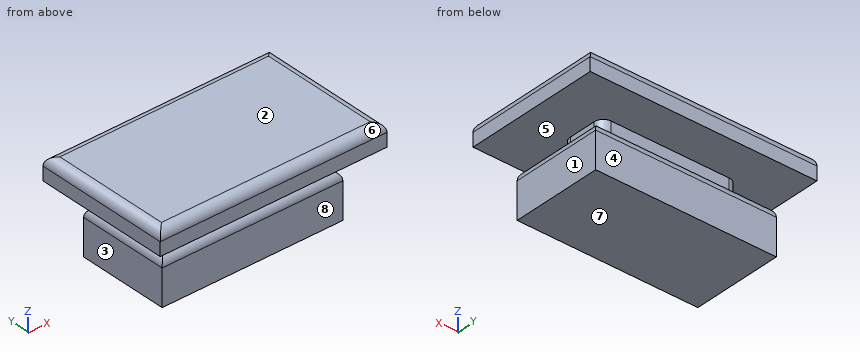
from build123d import *

# Parameters (mm, degrees)
F0_W     = 101.5923656523
F0_H     = 51.0535798967
F1_DEPTH = 25.4
F2_R     = 5.08
F3_W     = 76.4648839831
F3_H     = 25.6656967103
F4_DEPTH = 12.7
F5_R     = 5.08
F6_W     = 127.4997331202
F6_H     = 76.2346722186
F7_DEPTH = 12.7
F8_R     = 5.08


with BuildPart() as f1:
    # F0 (on Top) → F1 (new body)
    with BuildSketch(Plane.XY):
        with Locations((-14.3452938646, -5.9895161539)):
            Rectangle(F0_W, F0_H)
    extrude(amount=F1_DEPTH)

    # F2
    f2_edges = [f1.edges().sort_by_distance(p)[0] for p in [
        (-14.345294, -31.516306, 25.4),
        (-65.141477, -5.989516, 25.4),
        (-14.345294, 19.537274, 25.4),
        (36.450889, -5.989516, 25.4),
    ]]
    fillet(f2_edges, radius=F2_R)

    # F3 (on face) → F4 (join)
    with BuildSketch(Plane.XY.offset(25.4)):
        with Locations((-14.4407190382, -3.7901271135)):
            Rectangle(F3_W, F3_H)
    extrude(amount=F4_DEPTH)

    # F5
    f5_edges = [f1.edges().sort_by_distance(p)[0] for p in [
        (-52.673161, -16.622975, 31.75),
        (23.791723, -16.622975, 31.75),
        (-52.673161, 9.042721, 31.75),
        (23.791723, 9.042721, 31.75),
    ]]
    fillet(f5_edges, radius=F5_R)

    # F6 (on face) → F7 (join)
    with BuildSketch(Plane.XY.offset(38.1)):
        with Locations((-13.627236709, -6.3019637018)):
            Rectangle(F6_W, F6_H)
        with BuildLine():
            Line((-47.5931610298, 9.0427212417), (18.7117229533, 9.0427212417))
            ThreePointArc((18.7117229533, 9.0427212417), (22.3038254017, 7.5548236901), (23.7917229533, 3.9627212417))
            Line((23.7917229533, 3.9627212417), (23.7917229533, -11.5429754686))
            ThreePointArc((23.7917229533, -11.5429754686), (22.3038254017, -15.1350779171), (18.7117229533, -16.6229754686))
            Line((18.7117229533, -16.6229754686), (-47.5931610298, -16.6229754686))
            ThreePointArc((-47.5931610298, -16.6229754686), (-51.1852634782, -15.1350779171), (-52.6731610298, -11.5429754686))
            Line((-52.6731610298, -11.5429754686), (-52.6731610298, 3.9627212417))
            ThreePointArc((-52.6731610298, 3.9627212417), (-51.1852634782, 7.5548236901), (-47.5931610298, 9.0427212417))
        make_face(mode=Mode.SUBTRACT)
        with BuildLine():
            ThreePointArc((23.7917229533, 3.9627212417), (22.3038254017, 7.5548236901), (18.7117229533, 9.0427212417))
            Line((18.7117229533, 9.0427212417), (-47.5931610298, 9.0427212417))
            ThreePointArc((-47.5931610298, 9.0427212417), (-51.1852634782, 7.5548236901), (-52.6731610298, 3.9627212417))
            Line((-52.6731610298, 3.9627212417), (-52.6731610298, -11.5429754686))
            ThreePointArc((-52.6731610298, -11.5429754686), (-51.1852634782, -15.1350779171), (-47.5931610298, -16.6229754686))
            Line((-47.5931610298, -16.6229754686), (18.7117229533, -16.6229754686))
            ThreePointArc((18.7117229533, -16.6229754686), (22.3038254017, -15.1350779171), (23.7917229533, -11.5429754686))
            Line((23.7917229533, -11.5429754686), (23.7917229533, 3.9627212417))
        make_face()
    extrude(amount=F7_DEPTH)

    # F8
    f8_edges = [f1.edges().sort_by_distance(p)[0] for p in [
        (-13.627237, -44.4193, 50.8),
        (-77.377103, -6.301964, 50.8),
        (-13.627237, 31.815372, 50.8),
        (50.12263, -6.301964, 50.8),
    ]]
    fillet(f8_edges, radius=F8_R)


solid = f1.part
Input: part model. Units: mm. Frame: model coordinates. Face numbers are marked on the shaded views. A direction names the side the tool comes from. Give positions to 0.01 mm unless a question says otherwise; leave off trailing zeros. Loops run counter-clockwise (first coordinate to the right, second up) from the corner with the lowest first, then second, coordinate; pieces in that order, holes last. Notation, with made-up numbers: (63.5, 89.25) -> (86.5, 89.25) arc R19 cw to (86.5, 121.25) -> close; hole circle Ø1 at (48.25, 42). An arc over 180 degrees is marked (long way). Answer as a JSON object with one key per item and string values. Group by question number.
Item 1: Cut plane D-D, the plane y = -6. Return the cut outline in (x, z), and give its area (3 significant figures).
Item 2: Reachability of the marked faces 1, 2, 3 and 4 from +Z, -Z, +X, -X, +Y, -Y: full face, straight path, thin tool, end or side. Return the list, or none.
Item 3: Cut plane A-A, the plane y = 11. Return the cut outline in (x, z).
Item 4: Cut plane B-B, the plane z = 28.5. Return the cut outline in (x, y), and give its area (3 significant figures).
Item 5: Pin query (flat end, axial travel): P1, Ø10, axis at x = -2, z = 12.5, coming from the -Y side; P2, Ø10, axis at y = -8, z = 13, coming from the +X side; P3, Ø1.5, axis at x = -50.5, z = 24.5, coming from the -Y side; P4, Ø10, axis at x = 23.5, z = 35.5, coming from the +Y side. Return the tip coordinate at first contact, or that it passes through.
Item 6: Pull-direction query (Z, two-part tool) for the marked faces 5, 6, 7 and 8; classes: released by +Z, released by -Z, zero draft, split by the parting line, or undercut.
Item 7: Line query: probe 1 along Z at (x, y) = (27, -18); probe 2 along Y at (x, z) = (-8, 27.5); probe 3 along X at (y, z) = (-12, 20). Output: solid intervals per line, ascending.
Item 8: Cut plane C-C, the plane x = -1. Return the cut outline in (y, z), and give its area (3 significant figures).
Checks:
{
 "1": {"outline": "(-77.38, 38.1) -> (-52.67, 38.1) -> (-52.67, 25.4) -> (-60.06, 25.4) arc R5.08 ccw to (-65.14, 20.32) -> (-65.14, 0) -> (36.45, 0) -> (36.45, 20.32) arc R5.08 ccw to (31.37, 25.4) -> (23.79, 25.4) -> (23.79, 38.1) -> (50.12, 38.1) -> (50.12, 45.72) arc R5.08 ccw to (45.04, 50.8) -> (-72.3, 50.8) arc R5.08 ccw to (-77.38, 45.72) -> close", "area": "5,150 mm²"},
 "2": {"face 1": "-Z, +X, +Y, -Y", "face 2": "+Z, +X, -X, +Y, -Y", "face 3": "-Z, -X, +Y, -Y", "face 4": "-Z, +X, -X, +Y"},
 "3": {"outline": "(-77.38, 38.1) -> (50.12, 38.1) -> (50.12, 45.72) arc R5.08 ccw to (45.04, 50.8) -> (-72.3, 50.8) arc R5.08 ccw to (-77.38, 45.72) -> close; (-65.14, 0) -> (36.45, 0) -> (36.45, 20.32) arc R5.08 ccw to (31.37, 25.4) -> (-60.06, 25.4) arc R5.08 ccw to (-65.14, 20.32) -> close"},
 "4": {"outline": "(-52.67, -11.54) arc R5.08 ccw to (-47.59, -16.62) -> (18.71, -16.62) arc R5.08 ccw to (23.79, -11.54) -> (23.79, 3.96) arc R5.08 ccw to (18.71, 9.04) -> (-47.59, 9.04) arc R5.08 ccw to (-52.67, 3.96) -> close", "area": "1,940 mm²"},
 "5": {"P1": "stops at y = -31.52", "P2": "stops at x = 36.45", "P3": "stops at y = -30.18", "P4": "stops at y = 31.82"},
 "6": {"face 5": "undercut", "face 6": "released by +Z", "face 7": "released by -Z", "face 8": "zero draft"},
 "7": {"probe 1": "z = 0 to 25.4, 38.1 to 50.8", "probe 2": "y = -16.62 to 9.04", "probe 3": "x = -65.14 to 36.45"},
 "8": {"outline": "(-44.42, 38.1) -> (-16.62, 38.1) -> (-16.62, 25.4) -> (-26.44, 25.4) arc R5.08 ccw to (-31.52, 20.32) -> (-31.52, 0) -> (19.54, 0) -> (19.54, 20.32) arc R5.08 ccw to (14.46, 25.4) -> (9.04, 25.4) -> (9.04, 38.1) -> (31.82, 38.1) -> (31.82, 45.72) arc R5.08 ccw to (26.74, 50.8) -> (-39.34, 50.8) arc R5.08 ccw to (-44.42, 45.72) -> close", "area": "2,570 mm²"}
}
